Can you work these out from the model? Positions are in its coordinate system, mm. A direction names the side the tool comes from. Coordinates: 2 decimals unless noted, no trailing zeros. Loops run counter-clockwise (first coordinate to the right, second up) from the corner with the lowest first, then second, coordinate; pieces in that order, holes last.
```python
from build123d import *

# Parameters (mm, degrees)
SKETCH1_R           = 5
BOSS_EXTRUDE2_DEPTH = 4
CUT_EXTRUDE1_REACH  = 53.96


with BuildPart() as part:
    # Sketch1 → Boss-Extrude2 (new body)
    with BuildSketch(Plane.XY):
        with BuildLine():
            Line((10.16, 6.35), (10.16, -10.16))
            Line((10.16, -10.16), (6.16, -10.16))
            Line((6.16, -10.16), (6.16, -20.32))
            Line((6.16, -20.32), (10.16, -20.32))
            Line((10.16, -20.32), (10.16, -30.48))
            Line((10.16, -30.48), (6.16, -30.48))
            Line((6.16, -30.48), (6.16, -40.64))
            Line((6.16, -40.64), (10.16, -40.64))
            Line((10.16, -40.64), (10.16, -50.8))
            Line((10.16, -50.8), (6.062743352, -50.8))
            ThreePointArc((6.062743352, -50.8), (4.123604466, -50.269609791), (2.72436074, -48.826110437))
            Line((2.72436074, -48.826110437), (-9.688382612, -26.25748616))
            ThreePointArc((-9.688382612, -26.25748616), (-10.040212579, -25.36923179), (-10.16, -24.421375723))
            Line((-10.16, -24.421375723), (-10.16, 0))
            ThreePointArc((-10.16, 0), (-7.184204897, 7.184204897), (0, 10.16))
            Line((0, 10.16), (6.35, 10.16))
            ThreePointArc((6.35, 10.16), (9.044076836, 9.044076836), (10.16, 6.35))
        make_face()
        Circle(SKETCH1_R, mode=Mode.SUBTRACT)
    extrude(amount=BOSS_EXTRUDE2_DEPTH)

    # Sketch2 → Cut-Extrude1 (cut, up to next)
    with BuildSketch(Plane.XY.offset(4), mode=Mode.PRIVATE) as cut_extrude1_sk1:
        with BuildLine():
            Line((-6.124879753, -22.361389348), (-0.222794204, -33.092453983))
            ThreePointArc((-0.222794204, -33.092453983), (1.205952022, -33.71048803), (2.16, -32.480417171))
            Line((2.16, -32.480417171), (2.16, -21.749352536))
            ThreePointArc((2.16, -21.749352536), (1.788025612, -20.851326924), (0.89, -20.479352536))
            Line((0.89, -20.479352536), (-5.012085549, -20.479352536))
            ThreePointArc((-5.012085549, -20.479352536), (-6.105288813, -21.102972907), (-6.124879753, -22.361389348))
        make_face()
    cut_extrude1_tool1 = extrude(cut_extrude1_sk1.sketch, amount=-CUT_EXTRUDE1_REACH, mode=Mode.PRIVATE) & part.part
    add(cut_extrude1_tool1.solids().sort_by_distance((-1.019639, -25.736268, 4))[0], mode=Mode.SUBTRACT)


solid = part.part
```
Item 1: We'd pull the mould along X, two halves only. Please class faces 1 (the face through (6.16, -35, 2)), 2 (the face through (-6.096, -21.087, 2.028)), 3 (the face through (0, -13, 4)), 4 (the face through (-3.215, -27.652, 2.028)): +X half, -X half, draft (parallel to the pull), parting line (faces both ways), or undercut.
Results are:
face 1: +X half
face 2: undercut
face 3: draft
face 4: undercut
Item 2: Suppose I cut it at D-D, the plane x = 8. Please give me the cut outline in (y, z), plus the area to 3 significant figures.
Results are:
outline: (-50.8, 0) - (-40.64, 0) - (-40.64, 4) - (-50.8, 4) - close; (-30.48, 0) - (-20.32, 0) - (-20.32, 4) - (-30.48, 4) - close; (-10.16, 0) - (9.78, 0) - (9.78, 4) - (-10.16, 4) - close
area: 161 mm2
Item 3: Suppose I cut it at C-C, the plane x = 4. Please give me the cut outline in (y, z), plus the area to 3 significant figures.
Results are:
outline: (-50.19, 0) - (-3, 0) - (-3, 4) - (-50.19, 4) - close; (3, 0) - (10.16, 0) - (10.16, 4) - (3, 4) - close
area: 217 mm2
Item 4: Suppose I cut it at B-B, the plane y = -23. Please give me the cut outline in (x, z).
Results are:
outline: (-10.16, 0) - (-5.77, 0) - (-5.77, 4) - (-10.16, 4) - close; (2.16, 0) - (10.16, 0) - (10.16, 4) - (2.16, 4) - close
Item 5: I'm going to push flat-ended pins straight in: P1, Ø2, axis at x = -1.5, z = 3, coming from the +Y side; P2, Ø9, axis at x = 0, y = 0, coming from the -Z side. Where does each tip first touch, or does it pass through?
Results are:
P1: stops at y = 10.15
P2: passes through
Item 6: I need wall thicknesses on line 1 along Y through (x, z) = (0, 2.4); line 2 along Y through (x, z) = (7, 1.95); line 3 along X through (y, z) = (-33.5, 0.7) (3 decimals). Which ranges of each line are inside material? Lowest first, please.
Results are:
line 1: y = -43.87 to -33.39, -20.48 to -5, 5 to 10.16
line 2: y = -50.8 to -40.64, -30.48 to -20.32, -10.16 to 10.1
line 3: x = -5.705 to 0.133, 1.647 to 6.16
Item 7: On a 3-axis mill with a long thin cutter (end or side, diameter ignored), from which of +Z, -Z, +X, -X, +Y, -Y can I reach the whole of each face in a straight line? I mean faces 5 (the face through (-3.395, -37.7, 1.972)), 6 (the face through (1.183, -33.716, 2.028)), 7 (the face through (8, -40.64, 2)). Say none if no direction works.
Results are:
face 5: +Z, -Z, -X, -Y
face 6: +Z, -Z
face 7: +Z, -Z, +X
Item 8: Suppose I cut it at A-A, the plane z = 2.15. Please give me the cut outline in (x, y).
Results are:
outline: (-10.16, -24.42) arc R3.81 ccw to (-9.69, -26.26) - (2.72, -48.83) arc R3.81 ccw to (6.06, -50.8) - (10.16, -50.8) - (10.16, -40.64) - (6.16, -40.64) - (6.16, -30.48) - (10.16, -30.48) - (10.16, -20.32) - (6.16, -20.32) - (6.16, -10.16) - (10.16, -10.16) - (10.16, 6.35) arc R3.81 ccw to (6.35, 10.16) - (0, 10.16) arc R10.16 ccw to (-10.16, 0) - close; hole (-6.12, -22.36) - (-0.22, -33.09) arc R1.27 ccw to (2.16, -32.48) - (2.16, -21.75) arc R1.27 ccw to (0.89, -20.48) - (-5.01, -20.48) arc R1.27 ccw to start; hole circle Ø10 at (0, 0)
